from build123d import *

# Parameters (mm, degrees)
SKETCH1_R           = 10
BOSS_EXTRUDE1_DEPTH = 5


with BuildPart() as part:
    # Sketch1 → Boss-Extrude1 (new, symmetric)
    with BuildSketch(Plane.XY):
        with BuildLine():
            Line((-11.587303396, 53.12), (-24.140215409, 6.5))
            ThreePointArc((-24.140215409, 6.5), (-24.936514863, 1.780512988), (-24.81883517, -3.004233816))
            ThreePointArc((-24.81883517, -3.004233816), (-30.762049538, -19.776348187), (-47.717387131, -25.174694658))
            ThreePointArc((-47.717387131, -25.174694658), (-61.713032142, -49.370425713), (-35.03522611, -41.027395935))
            ThreePointArc((-35.03522611, -41.027395935), (-26.046643252, -25.670606045), (-8.378996809, -23.554031767))
            ThreePointArc((-8.378996809, -23.554031767), (0, -25), (8.378996809, -23.554031767))
            ThreePointArc((8.378996809, -23.554031767), (26.046643252, -25.670606045), (35.03522611, -41.027395935))
            ThreePointArc((35.03522611, -41.027395935), (61.713032142, -49.370425713), (47.717387131, -25.174694658))
            ThreePointArc((47.717387131, -25.174694658), (30.762049538, -19.776348187), (24.81883517, -3.004233816))
            ThreePointArc((24.81883517, -3.004233816), (24.936514863, 1.780512988), (24.140215409, 6.5))
            Line((24.140215409, 6.5), (11.587303396, 53.12))
            ThreePointArc((11.587303396, 53.12), (0, 62), (-11.587303396, 53.12))
        make_face()
        with Locations((50, -40)):
            Circle(SKETCH1_R, mode=Mode.SUBTRACT)
        with Locations(Location((-50, -40, 0), (0, 0, 180))):
            Circle(SKETCH1_R, mode=Mode.SUBTRACT)
        with BuildLine():
            Line((-4.769696007, 51.5), (-19.078784028, 6))
            ThreePointArc((-19.078784028, 6), (0, -20), (19.078784028, 6))
            Line((19.078784028, 6), (4.769696007, 51.5))
            ThreePointArc((4.769696007, 51.5), (0, 55), (-4.769696007, 51.5))
        make_face(mode=Mode.SUBTRACT)
    extrude(amount=BOSS_EXTRUDE1_DEPTH, both=True)


solid = part.part
Can you work these out from the model? Positions are in its coordinate system, mm. A direction names the side the tool comes from. Give positions to 0.01 mm unless a question says otherwise; leave off trailing zeros. Order: outer loops, then holes, each group sorted by start corner. A loop starts at its lowest first (then second) coordinate and runs counter-clockwise, first axis right, second up. Notation, with made-up numbers: M -7,-17 L 10,-17 A25 ccw 10,5 Z; hole C -12,49 d4. An arc over 180 degrees is marked long. Use a Markdown table: item, result. Add a question column.
Item 1: Suppose I cut it at B-B (y = 0). List the corners of the cut face in (x, z) for me.
Item 2: Suppose I cut it at D-D (y = -32). List the corners of the cut face in (x, z) for me, then the cut area to 3 significant figures.
Item 3: We'd pull the mould along Y, two halves only. Please class faces 3 (the cylindrical face through (-24.93, 1.85, 0.07)), 4 (the cylindrical face through (-62, -49, 0)), 5 (the flat face through (-17.776, 30.136, 0.07)), 6 (the cylindrical face through (-47.83, -30.24, -0.07)): +Y half, -Y half, draft (parallel to the pull), parting line (faces both ways), or undercut.
Item 4: For faces 1 (the flat face through (0, -22, 5)), 2 (the flat face through (12.024, 28.432, 0.07)), which set-ups out of +Z, -Z, +X, -X, +Y, -Y let a thin tool reach every point of the face, with its end or its side?
Item 5: Suppose I cut it at A-A (x = 0). List the corners of the cut face in (y, z) for me, then the cut area to 3 significant figures.
Item 6: Will these pins go through, and if not, where does the flat tip stop? pin 1 (1 mm diameter, centred on y = -1, z = 1.5, fed in from -X) (3 decimals); pin 2 (4 mm diameter, centred on y = 32.5, z = -3, fed in from +X); pin 3 (1 mm diameter, centred on y = -4.5, z = -1, fed in from +X); pin 4 (12 mm diameter, centred on x = -50, y = -40, fed in from +Z).
Item 7: Suppose I cut it at C-C (z = 3.5). List the corners of the cut face in (x, y) for me, then the cut area to 3 significant figures.
Item 8: If I drill on L1, parallel to X at y = 0, z = -2.5; L2, parallel to X at y = -39.5, z = 1.75; L3, parallel to X at y = -47.5, z = -3, over which ranges is the centre line in solid material (lowest first)? Write a range as [from, to].
Answer sheet:
| question | item | result |
|---|---|---|
| 1 | outline | M -25,-5 L -20,-5 L -20,5 L -25,5 Z; M 20,-5 L 25,-5 L 25,5 L 20,5 Z |
| 2 | outline | M -62.69,-5 L -56,-5 L -56,5 L -62.69,5 Z; M -44,-5 L -32.17,-5 L -32.17,5 L -44,5 Z; M 32.17,-5 L 44,-5 L 44,5 L 32.17,5 Z; M 56,-5 L 62.69,-5 L 62.69,5 L 56,5 Z |
| 2 | area | 370 mm² |
| 3 | face 3 | undercut |
| 3 | face 4 | parting line |
| 3 | face 5 | +Y half |
| 3 | face 6 | undercut |
| 4 | face 1 | +Z, +X, -X, +Y, -Y |
| 4 | face 2 | +Z, -Z |
| 5 | outline | M -25,-5 L -20,-5 L -20,5 L -25,5 Z; M 55,-5 L 62,-5 L 62,5 L 55,5 Z |
| 5 | area | 120 mm² |
| 6 | pin 1 | stops at x = -24.995 |
| 6 | pin 2 | stops at x = 17.68 |
| 6 | pin 3 | stops at x = 24.72 |
| 6 | pin 4 | passes through |
| 7 | outline | M -47.72,-25.17 A15 ccw long -35.04,-41.03 A20 cw -8.38,-23.55 A25 ccw 8.38,-23.55 A20 cw 35.04,-41.03 A15 ccw long 47.72,-25.17 A20 cw 24.82,-3 A25 ccw 24.14,6.5 L 11.59,53.12 A12 ccw -11.59,53.12 L -24.14,6.5 A25 ccw -24.82,-3 A20 cw Z; hole C -50,-40 d20; hole M -19.08,6 A20 ccw long 19.08,6 L 4.77,51.5 A5 ccw -4.77,51.5 Z; hole C 50,-40 d20 |
| 7 | area | 2,460 mm² |
| 8 | L1 | x = [-25, -20], [20, 25] |
| 8 | L2 | x = [-64.99, -59.99], [-40.01, -34.87], [34.87, 40.01], [59.99, 64.99] |
| 8 | L3 | x = [-62.99, -56.61], [-43.39, -37.01], [37.01, 43.39], [56.61, 62.99] |
